Read the model definition and answer for the solid it produces. Units are mm, in the model's axes. Coordinates: 2 decimals unless noted, no trailing zeros. Loops run counter-clockwise (first coordinate to the right, second up) from the corner with the lowest first, then second, coordinate; pieces in that order, holes last. Notation, with made-up numbers: (69, 49.5) - (78, 49.5) arc R12 cw to (78, 69.5) - close; hole circle Ø8 at (-15.5, 86). An arc over 180 degrees is marked (long way). Use one line per item in the form item = value. Start each with the question number.
1) Each of these flat-tipped pins is pushed along its axis until it touches: P1, Ø1.8, axis at x = 56, y = -8.5, coming from the -Z side; P2, Ø5, axis at x = -5.5, z = 8, coming from the -Y side. Where does it stop, or does it pass through?
2) Consider line 1 (Z direction, x = 61.65, y = -9); line 2 (X direction, y = -7.5, z = 7.25); line 3 (Y direction, x = -61.6, z = 8). Determine where each line is inside the solid, lowest interval first.
3) A cutting plane is placed at D-D (x = 1.5). Give the vertices of the cut face in (y, z), and give its area (3 significant figures).
4) A cutting plane is placed at B-B (z = 8). Give the vertices of the cut face in (x, y), and give its area (4 significant figures).
5) A cutting plane is placed at A-A (x = 45.79). Give the vertices of the cut face in (y, z).
6) A cutting plane is placed at C-C (y = -9). Give the vertices of the cut face in (x, z).
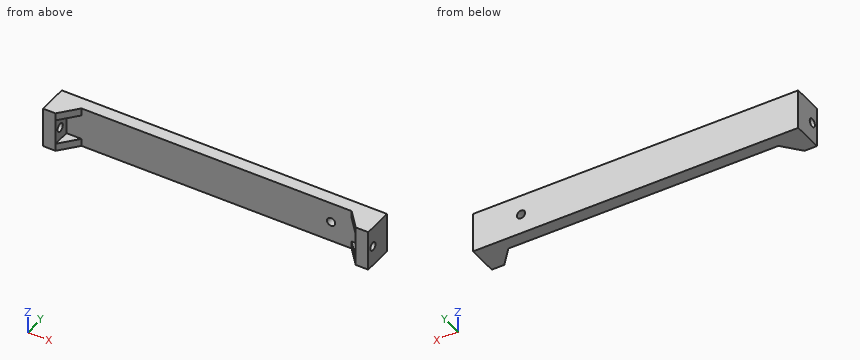
from build123d import *

# Parameters (mm, degrees)
EXTRUDE_2_DEPTH          = 16
SKETCH_3_R               = 1.65
CUT_EXTRUDE_1_DEPTH      = 126
CUT_EXTRUDE_1_DEPTH_BACK = 6
EXTRUDE_3_DEPTH          = 3
MIRROR_2_COPY_1_DEPTH    = 3
SKETCH_7_R               = 1.65
CUT_EXTRUDE_2_DEPTH      = 10


with BuildPart() as part:
    # 草图1 → 凸台-拉伸2 (new body)
    with BuildSketch(Plane.XY):
        Polygon((-65, 0), (65, 0), (65, -12), (60, -12), (60, -5), (-60, -5), (-60, -12), (-65, -12), align=None)
    extrude(amount=EXTRUDE_2_DEPTH)

    # 草图3 → 切除-拉伸1 (cut, two sides)
    with BuildSketch(Plane(origin=(-60, 0, 0), x_dir=(0, 0, -1), z_dir=(1, 0, 0))) as cut_extrude_1_sk:
        with Locations((-8, -9)):
            Circle(SKETCH_3_R)
    extrude(amount=CUT_EXTRUDE_1_DEPTH, mode=Mode.SUBTRACT)
    extrude(cut_extrude_1_sk.sketch, amount=-CUT_EXTRUDE_1_DEPTH_BACK, mode=Mode.SUBTRACT)

    # 草图4 → 凸台-拉伸3 (add)
    with BuildSketch(Plane(origin=(0, 0, 0), x_dir=(-1, 0, 0), z_dir=(0, 0, -1))):
        Polygon((54, -5), (60, -12), (60, -5), align=None)
    extrude_3 = extrude(amount=-EXTRUDE_3_DEPTH)

    # 镜向1: 凸台-拉伸3 across plane
    add(extrude_3.mirror(Plane.XY.offset(8)))

    # 镜向2: 凸台-拉伸3 across plane
    add(extrude_3.mirror(Plane(origin=(0, 0, 0), x_dir=(0, 0, 1), z_dir=(1, 0, 0))))

    # 镜向2 copy 1 sketch → 镜向2 copy 1 (add)
    with BuildSketch(Plane.XY.offset(16)):
        Polygon((54, -5), (60, -12), (60, -5), align=None)
    extrude(amount=-MIRROR_2_COPY_1_DEPTH)

    # 草图7 → 切除-拉伸2 (cut)
    with BuildSketch(Plane(origin=(0, 0, 0), x_dir=(1, 0, 0), z_dir=(0, 1, 0))):
        with Locations((45.79, -8)):
            Circle(SKETCH_7_R)
    extrude(amount=-CUT_EXTRUDE_2_DEPTH, mode=Mode.SUBTRACT)


solid = part.part
Found:
q1.P1 = 0
q1.P2 = -5
q2.line_1 = 0 to 6.35, 9.65 to 16
q2.line_2 = -65 to -60, 60 to 65
q2.line_3 = -12 to -10.65, -7.35 to 0
q3.outline = (-5, 0) - (0, 0) - (0, 16) - (-5, 16) - close
q3.area = 80.0 mm^2
q4.outline = (-65, -12) - (-60, -12) - (-60, -10.65) - (-65, -10.65) - close; (-65, -7.35) - (-60, -7.35) - (-60, -5) - (44.14, -5) - (44.14, 0) - (-65, 0) - close; (47.44, -5) - (60, -5) - (60, -7.35) - (65, -7.35) - (65, 0) - (47.44, 0) - close; (60, -12) - (65, -12) - (65, -10.65) - (60, -10.65) - close
q4.area = 670.5 mm^2
q5.outline = (-5, 0) - (0, 0) - (0, 6.35) - (-5, 6.35) - close; (-5, 9.65) - (0, 9.65) - (0, 16) - (-5, 16) - close
q6.outline = (-65, 0) - (-57.43, 0) - (-57.43, 3) - (-60, 3) - (-60, 6.35) - (-65, 6.35) - close; (-65, 9.65) - (-60, 9.65) - (-60, 13) - (-57.43, 13) - (-57.43, 16) - (-65, 16) - close; (57.43, 0) - (65, 0) - (65, 6.35) - (60, 6.35) - (60, 3) - (57.43, 3) - close; (57.43, 13) - (60, 13) - (60, 9.65) - (65, 9.65) - (65, 16) - (57.43, 16) - close
